Geometry: final body of the model. Coordinates: model frame, mm. A direction names the side the tool comes from. Give positions to 0.01 mm unless a question says otherwise; leave off trailing zeros. Order: outer loops, then holes, each group sorted by start corner. A loop starts at its lowest first (then second) coordinate and runs counter-clockwise, first axis right, second up. Notation, with made-up numbers: (47, -13) - (100, -13) arc R7 cw to (100, -2) - close; hole circle Ø8 at (25.5, -13.5). An arc over 180 degrees is marked (long way). One line per item, written item: value.
```python
from build123d import *

# Parameters (mm, degrees)
BOSS_EXTRUDE1_DEPTH = 50.8
SKETCH2_R           = 3.75
CUT_EXTRUDE1_DEPTH  = 50.8
SKETCH3_W           = 139.7
SKETCH3_H           = 38.1
CUT_EXTRUDE2_DEPTH  = 50.8
SKETCH4_R           = 5.5
CUT_EXTRUDE3_DEPTH  = 35
CHAMFER1_SIZE       = 2
CHAMFER2_SIZE       = 2


with BuildPart() as part:
    # Sketch1 → Boss-Extrude1 (new body)
    with BuildSketch(Plane.XY):
        with BuildLine():
            Line((-76.2, 10), (76.2, 10))
            ThreePointArc((76.2, 10), (86.2, 0), (76.2, -10))
            Line((76.2, -10), (-76.2, -10))
            ThreePointArc((-76.2, -10), (-86.2, 0), (-76.2, 10))
        make_face()
    extrude(amount=BOSS_EXTRUDE1_DEPTH)

    # Sketch2 → Cut-Extrude1 (cut)
    with BuildSketch(Plane.XY.offset(50.8)):
        with Locations((-76.2, 0)):
            Circle(SKETCH2_R)
        with Locations((76.2, 0)):
            Circle(SKETCH2_R)
    extrude(amount=-CUT_EXTRUDE1_DEPTH, mode=Mode.SUBTRACT)

    # Sketch3 → Cut-Extrude2 (cut)
    with BuildSketch(Plane(origin=(0, 10, 0), x_dir=(1, 0, 0), z_dir=(0, 1, 0))):
        with Locations((0, -19.05)):
            Rectangle(SKETCH3_W, SKETCH3_H)
    extrude(amount=-CUT_EXTRUDE2_DEPTH, mode=Mode.SUBTRACT)

    # Sketch4 → Cut-Extrude3 (cut)
    with BuildSketch(Plane.XY.offset(50.8)):
        with Locations((-76.2, 0)):
            Circle(SKETCH4_R)
        with Locations((76.2, 0)):
            Circle(SKETCH4_R)
    extrude(amount=-CUT_EXTRUDE3_DEPTH, mode=Mode.SUBTRACT)

    # Chamfer1
    chamfer1_edges = [part.edges().sort_by_distance(p)[0] for p in [
        (86.2, 0, 50.8),
        (0, 10, 50.8),
        (-86.2, 0, 50.8),
        (0, -10, 50.8),
    ]]
    chamfer(chamfer1_edges, length=CHAMFER1_SIZE)

    # Chamfer2
    # the kernel refuses this chamfer: 2 mm, written as the material it takes off along each edge
    with BuildSketch(Plane(origin=(76.2, 0, 15.8), x_dir=(1, 0, 0), z_dir=(0, -1, 0))) as chamfer2_piece_1_section:
        Polygon((3.75, -CHAMFER2_SIZE), (3.75 + CHAMFER2_SIZE, 0), (3.75, 0), align=None)
    chamfer2_piece_1 = revolve(axis=Axis((76.2, 0, 15.8), (0, 0, 1)), mode=Mode.PRIVATE)
    chamfer2_piece_1 = chamfer2_piece_1 & Plane(origin=(76.2, 0, 14.674245927), x_dir=(1, 0, 0), z_dir=(0, 0, 1)) * Cylinder(5.5, 23, mode=Mode.PRIVATE)
    add(chamfer2_piece_1, mode=Mode.SUBTRACT)
    with BuildSketch(Plane(origin=(-76.2, 0, 15.8), x_dir=(1, 0, 0), z_dir=(0, -1, 0))) as chamfer2_piece_2_section:
        Polygon((3.75, -CHAMFER2_SIZE), (3.75 + CHAMFER2_SIZE, 0), (3.75, 0), align=None)
    chamfer2_piece_2 = revolve(axis=Axis((-76.2, 0, 15.8), (0, 0, 1)), mode=Mode.PRIVATE)
    chamfer2_piece_2 = chamfer2_piece_2 & Plane(origin=(-76.2, 0, 14.674245927), x_dir=(1, 0, 0), z_dir=(0, 0, 1)) * Cylinder(5.5, 23, mode=Mode.PRIVATE)
    add(chamfer2_piece_2, mode=Mode.SUBTRACT)


solid = part.part
```
1) Mould query, pull axis Y, two halves, no side actions, for faces 1 (the face through (73.224, -2.282, 6.997)), 2 (the face through (85, 0, 50)), 3 (the face through (0, -10, 39)). Classes: released by +Y, released by -Y, zero draft, split by the parting line, or undercut.
Answers below:
face 1: undercut
face 2: split by the parting line
face 3: released by -Y
2) Section D-D, the plane z = 18.5. Return loops of the section in (x, y).
Answers below:
outline: (-76.2, -10) - (-69.85, -10) - (-69.85, 10) - (-76.2, 10) arc R10 ccw to start; (69.85, -10) - (76.2, -10) arc R10 ccw to (76.2, 10) - (69.85, 10) - close; hole circle Ø11 at (-76.2, 0); hole circle Ø11 at (76.2, 0)
3) Material intervals for line 1 along Y through (x, z) = (76.2, 26); line 2 along X through (y, z) = (-4.5, 41.5); line 3 along X through (y, z) = (3.5, 18.5), sorted ascending.
Answers below:
line 1: -10 to -5.5, 5.5 to 10
line 2: -85.13 to -79.36, -73.04 to 73.04, 79.36 to 85.13
line 3: -85.57 to -80.44, -71.96 to -69.85, 69.85 to 71.96, 80.44 to 85.57
4) First-contact query: pin 1 (6 mm diameter, centred on y = 3.5, z = 23, fed in from -X); pin 2 (6 mm diameter, centred on y = -4, z = 26.5, fed in from +X); pin 3 (12 mm diameter, centred on y = -3, z = 30, fed in from +X); pin 4 (2 mm diameter, centred on y = 3, z = 22, fed in from -X). Flat tips, straight axial feed; report the tip coordinate or a pass-through.
Answers below:
pin 1: x = -86.19
pin 2: x = 86.15
pin 3: x = 86.2
pin 4: x = -86
5) Section A-A, the plane z = 6.5. Return loops of the section in (x, y).
Answers below:
outline: (-76.2, -10) - (-69.85, -10) - (-69.85, 10) - (-76.2, 10) arc R10 ccw to start; (69.85, -10) - (76.2, -10) arc R10 ccw to (76.2, 10) - (69.85, 10) - close; hole circle Ø7.5 at (-76.2, 0); hole circle Ø7.5 at (76.2, 0)
6) Section C-C, the plane x = -35. Return loops of the section in (y, z).
Answers below:
outline: (-10, 38.1) - (10, 38.1) - (10, 48.8) - (8, 50.8) - (-8, 50.8) - (-10, 48.8) - close
7) Set-up query: faces 4 (the face through (69.85, 0, 19)), 5 (the face through (80, -2, 0)), 6 (the face through (-80.25, 3.72, 33.42)). Return all of +Z, -Z, +X, -X, +Y, -Y with unobstructed straight access to the full face (end or side cutting, diameter ignored); none if empty.
Answers below:
face 4: -Z, +Y, -Y
face 5: -Z, +X, -X, +Y, -Y
face 6: +Z
8) Section B-B, the plane y = 0. Return loops of the section in (x, z).
Answers below:
outline: (-86.2, 0) - (-79.95, 0) - (-79.95, 13.8) - (-81.7, 15.55) - (-81.7, 50.8) - (-84.2, 50.8) - (-86.2, 48.8) - close; (-72.45, 0) - (-69.85, 0) - (-69.85, 38.1) - (69.85, 38.1) - (69.85, 0) - (72.45, 0) - (72.45, 13.8) - (70.7, 15.55) - (70.7, 50.8) - (-70.7, 50.8) - (-70.7, 15.55) - (-72.45, 13.8) - close; (79.95, 0) - (86.2, 0) - (86.2, 48.8) - (84.2, 50.8) - (81.7, 50.8) - (81.7, 15.55) - (79.95, 13.8) - close
